Could you check a few things on this drawing? It's one solid part, dimensions in mm from its lowest x, y, z. Give positions to 0.01 mm unless a question says otherwise; leave off trailing zeros. Order: outer loops, then holes, each group sorted by start corner. A loop starts at its lowest first (then second) coordinate and runs counter-clockwise, first axis right, second up.
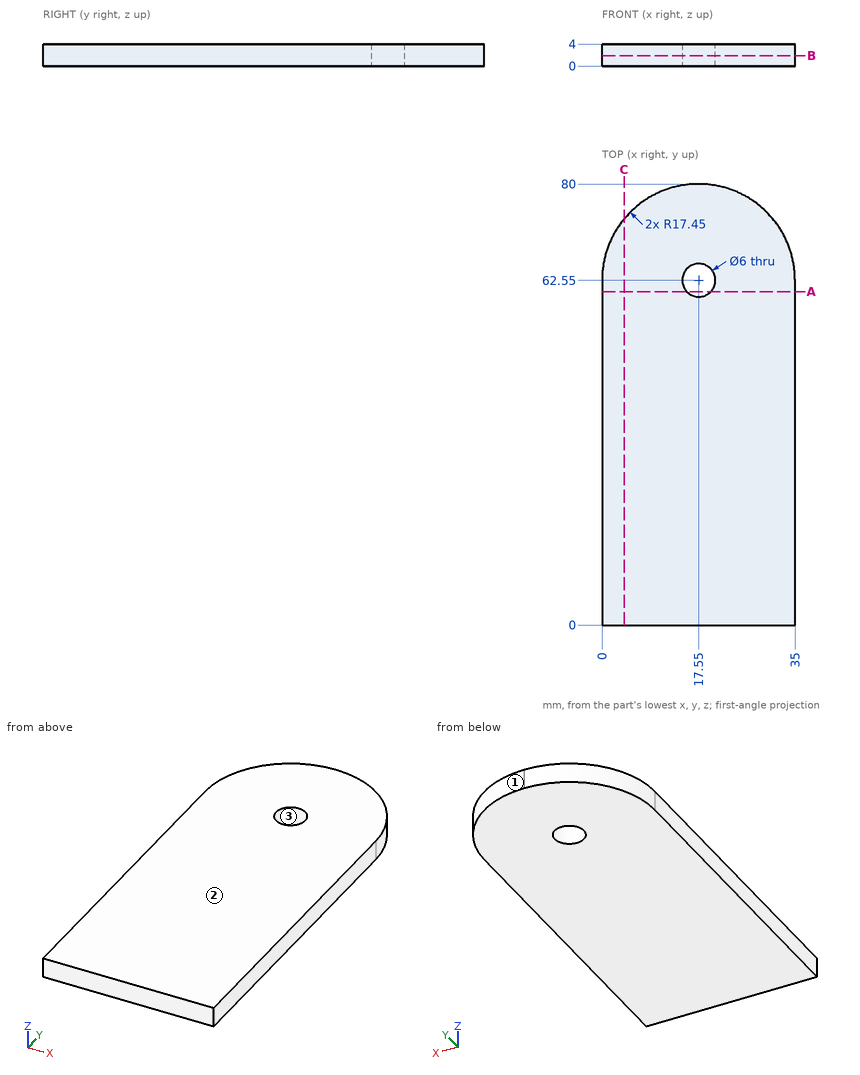
Item 1: Imagine slicing it at A-A on y = 60.5. List the corners of the cut face in (x, z) for me.
Findings:
outline: (0, 0) - (15.36, 0) - (15.36, 4) - (0, 4) - close; (19.74, 0) - (35, 0) - (35, 4) - (19.74, 4) - close
Item 2: Imagine slicing it at B-B on z = 1.9. List the corners of the cut face in (x, y) for me, then the cut area to 3 significant figures.
Findings:
outline: (0, 0) - (35, 0) - (35, 62.55) arc R17.45 ccw to (17.55, 80) - (17.45, 80) arc R17.45 ccw to (0, 62.55) - close; hole circle Ø6 at (17.55, 62.55)
area: 2,640 mm2
Item 3: Please list where these lines run through material, in increasing order: line 1 along Y through (x, z) = (17.55, 2.95); line 2 along Y through (x, z) = (16, 1.85); line 3 along X through (y, z) = (70, 3.1).
Findings:
line 1: y = 0 to 59.55, 65.55 to 80
line 2: y = 0 to 59.98, 65.12 to 79.94
line 3: x = 1.67 to 33.33
Item 4: Imagine slicing it at C-C on x = 4. List the corners of the cut face in (y, z) for me.
Findings:
outline: (0, 0) - (73.67, 0) - (73.67, 4) - (0, 4) - close
Item 5: We'd pull the mould along Y, two halves only. Please class the marked faces 1, 2 and 3: +Y half, -Y half, draft (parallel to the pull), parting line (faces both ways), or undercut.
Findings:
face 1: +Y half
face 2: draft
face 3: undercut
Item 6: For pin 1 (1.5 mm diameter, centred on x = 9, z = 1, fed in from +Y); pin 2 (2 mm diameter, centred on x = 24.5, z = 2, fed in from +Y), each with a flat end and sliding along its axis, tell me the tip position at first contact or that it passes through.
Findings:
pin 1: stops at y = 78.21
pin 2: stops at y = 78.95
